Read the model definition and answer for the solid it produces. Units are mm, in the model's axes. A direction names the side the tool comes from. Round coordinates to 2 decimals unless told otherwise and drop trailing zeros. Write each loop counter-clockwise with the first axis right and the second up, starting at its lowest first coordinate (ties: lowest second). Pieces come first, ordered by that corner, then holes. Notation, with made-up numbers: (33, 67) - (47, 67) arc R19 cw to (47, 74) - close; hole circle Ø11 at (-13, -7). An arc over 180 degrees is marked (long way). Use one line per item in the form item = value. Start each with the question number.
1) For a pull along X with two mould halves and no side action, classify faces 3 (the face through (30.584, 0, 2)), 4 (the face through (9.35, 7.17, 6.96)), 5 (the face through (0, 5, 0)), 6 (the face through (-0.06, -11.07, 8.03)) as released by +X, released by -X, zero draft, split by the parting line, or undercut.
2) Consider line 1 along X through (y, z) = (0, 3); line 2 along Y through (x, z) = (0, 3); line 3 along Z through (x, y) = (-20, -13). Determine where each line is inside the solid, lowest interval first. Write a range as from..to.
3) Each of these flat-tipped pins is pushed along its axis until it touches: pin 1 (2 mm diameter, centred on y = -2, z = 7.5, fed in from +X); pin 2 (1.7 mm diameter, centred on x = 1.5, y = 7, fed in from +Z). Where does it stop, or does it pass through?
4) The part is cut by section B-B, the plane y = -1.5. Give the vertices of the cut face in (x, z), plus the area to 3 significant figures.
5) For faces 1 (the face through (-2.533, 6.41, 8.028)), 2 (the face through (0, -22.376, 2)), determine the directions among +Z, -Z, +X, -X, +Y, -Y from which every point of the face is accessible in a straight line to the end or side of a thin tool.
6) The part is cut by section D-D, the plane z = 1.5. Give the vertices of the cut face in (x, y), plus the area to 3 significant figures.
7) The part is cut by section A-A, the plane z = 7. Give the vertices of the cut face in (x, y), plus the area to 3 significant figures.
from build123d import *

# Parameters (mm, degrees)
ESQUISSE1_W             = 61.168999858
ESQUISSE1_H             = 44.751998484
ESQUISSE1_R             = 3.815511502
BOSS_EXTRU_2_DEPTH      = 4
BOSS_EXTRU_4_START      = 4
ESQUISSE2_R             = 11.783463465
BOSS_EXTRU_4_DEPTH      = 6
ENL_V_MAT_EXTRU_1_DEPTH = 4
ESQUISSE1_2_R           = 3.815511502
ENL_V_MAT_EXTRU_3_DEPTH = 40.193073087


with BuildPart() as part:
    # Esquisse1 → Boss.-Extru.2 (new body)
    with BuildSketch(Plane.XY):
        Rectangle(ESQUISSE1_W, ESQUISSE1_H)
        Circle(ESQUISSE1_R, mode=Mode.SUBTRACT)
    extrude(amount=BOSS_EXTRU_2_DEPTH)

    # Esquisse2 → Boss.-Extru.4 (add)
    with BuildSketch(Plane.XY.offset(BOSS_EXTRU_4_START)):
        with Locations(Location((0, 0, 0), (0, 0, 180))):
            Circle(ESQUISSE2_R)
    extrude(amount=BOSS_EXTRU_4_DEPTH)

    # Esquisse4 → Enl_v. mat.-Extru.1 (cut)
    with BuildSketch(Plane.XY.offset(10)):
        with BuildLine():
            Line((2.87019869, 2.302904251), (2.212319523, 10.306766943))
            ThreePointArc((2.212319523, 10.306766943), (-0.029730087, 11.070975118), (-2.223029733, 10.17641531))
            Line((-2.223029733, 10.17641531), (-2.870198645, 2.302904307))
            ThreePointArc((-2.870198645, 2.302904307), (-3.679865285, 0), (-2.870198645, -2.302904307))
            Line((-2.870198645, -2.302904307), (-2.223029733, -10.17641531))
            ThreePointArc((-2.223029733, -10.17641531), (-0.029730087, -11.070975118), (2.212319523, -10.306766943))
            Line((2.212319523, -10.306766943), (2.87019869, -2.302904251))
            ThreePointArc((2.87019869, -2.302904251), (3.679865285, 0), (2.87019869, 2.302904251))
        make_face()
    extrude(amount=-ENL_V_MAT_EXTRU_1_DEPTH, mode=Mode.SUBTRACT)

    # Esquisse1_2 → Enl_v. mat.-Extru.3 (cut, through all)
    with BuildSketch(Plane.XY):
        with Locations(Location((0, 0, 0), (0, 0, 138.351064991))):
            Circle(ESQUISSE1_2_R)
    extrude(amount=ENL_V_MAT_EXTRU_3_DEPTH, mode=Mode.SUBTRACT)


solid = part.part
Geometry results:
q1.face_3 = released by +X
q1.face_4 = split by the parting line
q1.face_5 = zero draft
q1.face_6 = undercut
q2.line_1 = -30.58..-3.82, 3.82..30.58
q2.line_2 = -22.38..-3.82, 3.82..22.38
q2.line_3 = 0..4
q3.pin_1 = 11.74
q3.pin_2 = 6
q4.outline = (-30.58, 0) - (-3.51, 0) - (-3.51, 10) - (-11.69, 10) - (-11.69, 4) - (-30.58, 4) - close; (3.51, 0) - (30.58, 0) - (30.58, 4) - (11.69, 4) - (11.69, 10) - (3.51, 10) - close
q4.area = 315 mm2
q5.face_1 = +Z
q5.face_2 = +Z, -Z, +X, -X, -Y
q6.outline = (-30.58, -22.38) - (30.58, -22.38) - (30.58, 22.38) - (-30.58, 22.38) - close; hole circle Ø7.63 at (0, 0)
q6.area = 2,690 mm2
q7.outline = circle Ø23.57 at (0, 0); hole (-2.85, -2.54) - (-2.22, -10.18) arc R3.38 ccw to (2.21, -10.31) - (2.85, -2.54) arc R3.82 ccw to (2.85, 2.54) - (2.21, 10.31) arc R3.38 ccw to (-2.22, 10.18) - (-2.85, 2.54) arc R3.82 ccw to start
q7.area = 317 mm2
